from build123d import *

# Parameters (mm, degrees)
F0_R     = 2.5
F1_DEPTH = 4
F2_W     = 12
F2_H     = 15
F3_DEPTH = 2.286


with BuildPart() as f1:
    # F0 (on Front) → F1 (new body)
    with BuildSketch(Plane.XZ):
        with BuildLine():
            Line((3.81, 3.81), (0, 3.81))
            ThreePointArc((0, 3.81), (-3.81, 0), (0, -3.81))
            Line((0, -3.81), (3.81, -3.81))
            Line((3.81, -3.81), (3.81, 3.81))
        make_face()
        Circle(F0_R, mode=Mode.SUBTRACT)
    extrude(amount=F1_DEPTH)

    # F2 (on face) → F3 (join)
    with BuildSketch(Plane.YZ.offset(3.81)):
        with Locations((-2, 0)):
            Rectangle(F2_W, F2_H)
    extrude(amount=F3_DEPTH)


solid = f1.part
Could you check a few things on this model? Use its own coordinates, in mm. A direction names the side the tool comes from. Give positions to 0.01 mm unless a question says otherwise; leave off trailing zeros. Write each loop counter-clockwise with the first axis right and the second up, starting at its lowest first coordinate (ties: lowest second). Pieces come first, ordered by that corner, then holes. Notation, with made-up numbers: (-14, 13.5) -> (-4, 13.5) arc R5 ccw to (-4, 21.5) -> close; hole circle Ø2 at (-38, 33.5). An arc over 180 degrees is marked (long way). Answer as CSV lines item,"result". Start each with the question number.
(1) If we section it at A-A, the plane z = 0: Write out the boundary of the cut face in (x, y), and give its area (3 significant figures).
(2) I'm going to push flat-ended pins straight in: pin 1 Ø5 at (x, y) = (-0.5, -1) entering from +Z; pin 2 Ø4 at (x, z) = (-1.5, 1.5) entering from -Y; pin 3 Ø4 at (x, y) = (1.5, -1.5) entering from -Z. Where does each tip first touch, or does it pass through?
(3) If we mould it in two halves opening along X, with no side actions, what happens to faces 1 (the face through (-3.81, -1.97, 0.08)), 2 (the face through (-0.54, -1.97, -2.44)), 3 (the face through (5, -2, 7.5))? For each: +X half, -X half, draft (parallel to the pull), parting line (faces both ways), or undercut.
(4) Please list where these lines run through material, in increasing order: line 1 (Z direction, x = 0, y = -1.25); line 2 (X direction, y = -5.75, z = -2.75); line 3 (Y direction, x = -2.25, z = 3).
(5) If we section it at C-C, the plane x = 2.25: Write out the boundary of the cut face in (y, z).
(6) Which directions (+Z, -Z, +X, -X, +Y, -Y) give clear straight access to the entire face, cutting with the end or side of a thin tool? Please do faces 4 (the face through (2, -2, 3.81)), 5 (the face through (2.5, 0, 0.9)), 6 (the face through (2, -2, -3.81)), 7 (the face through (2.5, -4, 0.9)).
(7) If we section it at D-D, the plane z = -3: Write out the boundary of the cut face in (x, y), and give its area (3 significant figures).
(8) If we section it at B-B, the plane y = -2.75: Write out the boundary of the cut face in (x, z), and give its area (3 significant figures).
Answer list:
1,outline,"(-3.81, -4) -> (-2.5, -4) -> (-2.5, 0) -> (-3.81, 0) -> close; (2.5, -4) -> (3.81, -4) -> (3.81, -8) -> (6.1, -8) -> (6.1, 4) -> (3.81, 4) -> (3.81, 0) -> (2.5, 0) -> close"
1,area,"37.9 mm^2"
2,pin 1,"z = 3.81"
2,pin 2,"y = -4"
2,pin 3,"z = -3.81"
3,face 1,"-X half"
3,face 2,"undercut"
3,face 3,"draft"
4,line 1,"-3.81 to -2.5, 2.5 to 3.81"
4,line 2,"3.81 to 6.1"
4,line 3,"-4 to 0"
5,outline,"(-4, -3.81) -> (0, -3.81) -> (0, -1.09) -> (-4, -1.09) -> close; (-4, 1.09) -> (0, 1.09) -> (0, 3.81) -> (-4, 3.81) -> close"
6,face 4,"+Z, -X, +Y, -Y"
6,face 5,"+Z, -Z, -X, +Y"
6,face 6,"-Z, -X, +Y, -Y"
6,face 7,"+Z, -Z, -X, -Y"
7,outline,"(-2.35, -4) -> (3.81, -4) -> (3.81, -8) -> (6.1, -8) -> (6.1, 4) -> (3.81, 4) -> (3.81, 0) -> (-2.35, 0) -> close"
7,area,"52.1 mm^2"
8,outline,"(0, -3.81) -> (3.81, -3.81) -> (3.81, -7.5) -> (6.1, -7.5) -> (6.1, 7.5) -> (3.81, 7.5) -> (3.81, 3.81) -> (0, 3.81) arc R3.81 ccw to start; hole circle Ø5 at (0, 0)"
8,area,"66.5 mm^2"
